```python
from build123d import *

# Parameters (mm, degrees)
BOSS_EXTRUDE1_DEPTH     = 5.08
SKETCH1_3_W             = 5.08
SKETCH1_3_H             = 20.32
BOSS_EXTRUDE2_DEPTH     = 12.7
CUT_EXTRUDE1_DEPTH      = 94.22598993
CUT_EXTRUDE1_DEPTH_BACK = 94.22598993
SKETCH2_R               = 1.5


with BuildPart() as part:
    # Sketch1 → Boss-Extrude1 (new body)
    with BuildSketch(Plane.XY):
        with BuildLine():
            Line((90.0938, 10.16), (90.0938, 20.32))
            Line((90.0938, 20.32), (5.08, 20.32))
            Line((5.08, 20.32), (5.08, 10.16))
            Line((5.08, 10.16), (31.4947, 10.16))
            ThreePointArc((31.4947, 10.16), (32.5869, 11.2522), (33.6791, 10.16))
            Line((33.6791, 10.16), (61.4947, 10.16))
            ThreePointArc((61.4947, 10.16), (62.5869, 11.2522), (63.6791, 10.16))
            Line((63.6791, 10.16), (90.0938, 10.16))
        make_face()
        with BuildLine():
            Line((90.0938, 0), (90.0938, 10.16))
            Line((90.0938, 10.16), (63.6791, 10.16))
            ThreePointArc((63.6791, 10.16), (62.5869, 9.0678), (61.4947, 10.16))
            Line((61.4947, 10.16), (33.6791, 10.16))
            ThreePointArc((33.6791, 10.16), (32.5869, 9.0678), (31.4947, 10.16))
            Line((31.4947, 10.16), (5.08, 10.16))
            Line((5.08, 10.16), (5.08, 0))
            Line((5.08, 0), (90.0938, 0))
        make_face()
    extrude(amount=BOSS_EXTRUDE1_DEPTH)

    # Sketch1_3 → Boss-Extrude2 (add)
    with BuildSketch(Plane.XY):
        with Locations((92.6338, 10.16)):
            Rectangle(SKETCH1_3_W, SKETCH1_3_H)
        with Locations((2.54, 10.16)):
            Rectangle(SKETCH1_3_W, SKETCH1_3_H)
    extrude(amount=BOSS_EXTRUDE2_DEPTH)

    # Sketch2 → Cut-Extrude1 (cut, two sides: drawn at the far end of the back side and taken through both)
    with BuildSketch(Plane.ZY.offset(-90.0938).offset(-CUT_EXTRUDE1_DEPTH_BACK)):
        with Locations(Location((8.89, 16.51, 0), (0, 0, 90))):
            Circle(SKETCH2_R)
        with Locations(Location((8.89, 3.81, 0), (0, 0, 90))):
            Circle(SKETCH2_R)
    extrude(amount=CUT_EXTRUDE1_DEPTH + CUT_EXTRUDE1_DEPTH_BACK, mode=Mode.SUBTRACT)


solid = part.part
```
The listing builds one solid part. Answer for the finished solid, in the listing's coordinates (mm). A direction names the side the tool comes from. Give positions to 0.01 mm unless a question says otherwise; leave off trailing zeros. Order: outer loops, then holes, each group sorted by start corner. A loop starts at its lowest first (then second) coordinate and runs counter-clockwise, first axis right, second up. Notation, with made-up numbers: M 35,-24.5 L 75,-24.5 A17 ccw 75,3.5 Z; hole C -25,24.25 d4. An arc over 180 degrees is marked long. Put each result on its own line as item: value. Start each with the question number.
Item 1: The part is cut by section C-C, the plane y = 16.51. Determine the outline of the cut face in (x, z), and give its area (3 significant figures).
Item 2: Which of the six approach directions +Z, -Z, +X, -X, +Y, -Y give full straight-line access (tool end or side, diameter ignored) to faces 1 (the face through (90.094, 10, 9)), 2 (the face through (47, 20.32, 3))?
Item 3: The part is cut by section D-D, the plane x = 41. Determine the outline of the cut face in (y, z), and give its area (3 significant figures).
Item 4: The part is cut by section B-B, the plane z = 8.89. Determine the outline of the cut face in (x, y), and give its area (3 significant figures).
Item 5: The part is cut by section A-A, the plane y = 10.16. Determine the outline of the cut face in (x, z), and give its area (3 significant figures).
Item 6: For a pull along Y with two mould halves and no side action, classify faces 3 (the face through (2.58, 15.01, 8.82)), 4 (the face through (47, 0, 3)), 5 (the face through (5.08, 10, 9)) as +Y half, -Y half, draft (parallel to the pull), parting line (faces both ways), or undercut.
Item 7: Find the intervals of material crossed by line 1 along X through (y, z) = (10.16, 2.1); line 2 along X through (y, z) = (2.5, 6); line 3 along Z through (x, y) = (92.4, 16.51), in increasing order.
Item 8: Flat-ended cylindrical pins translate along their axes: P1, Ø5, axis at y = 12.5, z = 4, coming from the -X side; P2, Ø2.5, axis at x = 62.59, y = 10.16, coming from the +Z side; P3, Ø1, axis at x = 70, z = 6.5, coming from the +Y side. Find the tip coordinate at first contact, or state that the pin passes through.
Answer key:
1. outline: M 0,0 L 95.17,0 L 95.17,7.39 L 90.09,7.39 L 90.09,5.08 L 5.08,5.08 L 5.08,7.39 L 0,7.39 Z; M 0,10.39 L 5.08,10.39 L 5.08,12.7 L 0,12.7 Z; M 90.09,10.39 L 95.17,10.39 L 95.17,12.7 L 90.09,12.7 Z
1. area: 530 mm²
2. face 1: +Z, +Y, -Y
2. face 2: +Z, -Z, +X, -X, +Y
3. outline: M 0,0 L 20.32,0 L 20.32,5.08 L 0,5.08 Z
3. area: 103 mm²
4. outline: M 0,0 L 5.08,0 L 5.08,2.31 L 0,2.31 Z; M 0,5.31 L 5.08,5.31 L 5.08,15.01 L 0,15.01 Z; M 0,18.01 L 5.08,18.01 L 5.08,20.32 L 0,20.32 Z; M 90.09,0 L 95.17,0 L 95.17,2.31 L 90.09,2.31 Z; M 90.09,5.31 L 95.17,5.31 L 95.17,15.01 L 90.09,15.01 Z; M 90.09,18.01 L 95.17,18.01 L 95.17,20.32 L 90.09,20.32 Z
4. area: 145 mm²
5. outline: M 0,0 L 31.49,0 L 31.49,5.08 L 5.08,5.08 L 5.08,12.7 L 0,12.7 Z; M 33.68,0 L 61.49,0 L 61.49,5.08 L 33.68,5.08 Z; M 63.68,0 L 95.17,0 L 95.17,12.7 L 90.09,12.7 L 90.09,5.08 L 63.68,5.08 Z
5. area: 539 mm²
6. face 3: undercut
6. face 4: -Y half
6. face 5: draft
7. line 1: x = 0 to 31.49, 33.68 to 61.49, 63.68 to 95.17
7. line 2: x = 0 to 5.08, 90.09 to 95.17
7. line 3: z = 0 to 7.39, 10.39 to 12.7
8. P1: stops at x = 0
8. P2: stops at z = 5.08
8. P3: passes through
